```python
from build123d import *

# Parameters (mm, degrees)
F0_R     = 36.5
F0_R_2   = 31.5
F1_DEPTH = 7
F0_R_3   = 39.25
F2_DEPTH = 2
F3_R     = 18.5
F3_R_2   = 16
F4_DEPTH = 6
F5_DEPTH = 25
F7_DEPTH = 5


with BuildPart() as f1:
    # F0 (on Top) → F1 (new body)
    with BuildSketch(Plane.XY):
        Circle(F0_R)
        Circle(F0_R_2, mode=Mode.SUBTRACT)
        Circle(F0_R_2)
    extrude(amount=F1_DEPTH)

    # F0 (on Top) → F2 (join)
    with BuildSketch(Plane.XY):
        Circle(F0_R_3)
        Circle(F0_R, mode=Mode.SUBTRACT)
        Circle(F0_R)
        Circle(F0_R_2, mode=Mode.SUBTRACT)
    extrude(amount=F2_DEPTH)

    # F3 (on face) → F4 (cut)
    with BuildSketch(Plane.XY.offset(7)):
        Circle(F3_R)
        Circle(F3_R_2, mode=Mode.SUBTRACT)
        Circle(F3_R_2)
    extrude(amount=-F4_DEPTH, mode=Mode.SUBTRACT)

    # F3 (on face) → F5 (cut)
    with BuildSketch(Plane.XY.offset(7)):
        Circle(F3_R_2)
    extrude(amount=-F5_DEPTH, mode=Mode.SUBTRACT)

    # F6 (on face) → F7 (cut)
    with BuildSketch(Plane.XY.offset(7)):
        Polygon((17.3205080757, -6.5), (40, -6.5), (40, 6.5), (17.3205080757, 6.5), (-17.3205080757, 6.5), (-40, 6.5), (-40, -6.5), (-17.3205080757, -6.5), align=None)
        with BuildLine():
            Line((-35.9165699921, 6.5), (-17.3205080757, 6.5))
            Line((-17.3205080757, 6.5), (-34.1728943115, 12.8243243243))
            ThreePointArc((-34.1728943115, 12.8243243243), (-35.1871073141, 9.7014163331), (-35.9165699921, 6.5))
        make_face()
        with BuildLine():
            Line((-34.1728943115, -12.8243243243), (-17.3205080757, -6.5))
            Line((-17.3205080757, -6.5), (-35.9165699921, -6.5))
            ThreePointArc((-35.9165699921, -6.5), (-35.1871073141, -9.7014163331), (-34.1728943115, -12.8243243243))
        make_face()
        with BuildLine():
            Line((35.9165699921, -6.5), (17.3205080757, -6.5))
            Line((17.3205080757, -6.5), (34.1728943115, -12.8243243243))
            ThreePointArc((34.1728943115, -12.8243243243), (35.1871073141, -9.7014163331), (35.9165699921, -6.5))
        make_face()
        with BuildLine():
            Line((34.1728943115, 12.8243243243), (17.3205080757, 6.5))
            Line((17.3205080757, 6.5), (35.9165699921, 6.5))
            ThreePointArc((35.9165699921, 6.5), (35.1871073141, 9.7014163331), (34.1728943115, 12.8243243243))
        make_face()
    extrude(amount=-F7_DEPTH, mode=Mode.SUBTRACT)


solid = f1.part
```
Part model, mm, in its own coordinate system. A direction names the side the tool comes from. Round coordinates to 2 decimals unless told otherwise and drop trailing zeros. Loops run counter-clockwise (first coordinate to the right, second up) from the corner with the lowest first, then second, coordinate; pieces in that order, holes last. Notation, with made-up numbers: (41.25, 20) -> (46.25, 20) arc R22 ccw to (46.25, 41) -> close; hole circle Ø4 at (-0.75, -33.5). An arc over 180 degrees is marked (long way). Use one line per item in the form item = value. Start each with the question number.
Item 1: Band-saw the part on B-B (x = 0). List the corners of the cut face in (y, z), plus the area to 3 significant figures.
Item 2: Band-saw the part on D-D (y = -25.5). List the corners of the cut face in (x, z).
Item 3: Tool access for faces 4 (the flat face through (-18, 6, 2)), 5 (the cylindrical face through (0.619, 36.495, 4.465)), 6 (the flat face through (25.63, -9.62, 4.54)): list every direction of +Z, -Z, +X, -X, +Y, -Y with a clear straight run to the whole face (end or side of a thin tool).
Item 4: Drop flat-ended pins along their axis: pin 1 Ø4 at (y, z) = (14.5, 1.5) entering from -X; pin 2 Ø4 at (x, z) = (-29.5, 6) entering from -Y; pin 3 Ø2 at (y, z) = (-28.5, 1) entering from -X. Give the stop position or say it passes through.
Item 5: Band-saw the part on A-A (z = 4.5). List the corners of the cut face in (x, y).
Item 6: Drill centre lines: line 1 along Y through (x, z) = (0, 0.65); line 2 along Y through (x, z) = (0, 3.25); line 3 along Z through (x, y) = (35, 3.5). Where is each one in solid material? Low to high.
Item 7: Band-saw the part on C-C (y = 0). List the corners of the cut face in (x, z), plus the area to 3 significant figures.
Item 8: Two-plate mould, pull along X, no slides. Class faces 1 (the flat face through (-25.865, -9.706, 4.535)), 2 (the flat face through (-6, 15, 1)), 3 (the flat face through (0, 22, 7)): released by +X, released by -X, zero draft, split by the parting line, or undercut.
Data:
q1.outline = (-39.25, 0) -> (-16, 0) -> (-16, 1) -> (-18.5, 1) -> (-18.5, 7) -> (-36.5, 7) -> (-36.5, 2) -> (-39.25, 2) -> close; (16, 0) -> (39.25, 0) -> (39.25, 2) -> (36.5, 2) -> (36.5, 7) -> (18.5, 7) -> (18.5, 1) -> (16, 1) -> close
q1.area = 268 mm^2
q2.outline = (-29.84, 0) -> (29.84, 0) -> (29.84, 2) -> (26.12, 2) -> (26.12, 7) -> (-26.12, 7) -> (-26.12, 2) -> (-29.84, 2) -> close
q3.face_4 = +Z
q3.face_5 = +Z, +Y
q3.face_6 = +Z, +X
q4.pin_1 = -37.21
q4.pin_2 = -24
q4.pin_3 = -28.01
q5.outline = (-34.17, -12.82) arc R36.5 ccw to (34.17, -12.82) -> (17.32, -6.5) arc R18.5 cw to (-17.32, -6.5) -> close; (-34.17, 12.82) -> (-17.32, 6.5) arc R18.5 cw to (17.32, 6.5) -> (34.17, 12.82) arc R36.5 ccw to start
q6.line_1 = -39.25 to -16, 16 to 39.25
q6.line_2 = -36.5 to -18.5, 18.5 to 36.5
q6.line_3 = 0 to 2
q7.outline = (-39.25, 0) -> (-16, 0) -> (-16, 1) -> (-18.5, 1) -> (-18.5, 2) -> (-39.25, 2) -> close; (16, 0) -> (39.25, 0) -> (39.25, 2) -> (18.5, 2) -> (18.5, 1) -> (16, 1) -> close
q7.area = 88.0 mm^2
q8.face_1 = released by -X
q8.face_2 = undercut
q8.face_3 = zero draft
